Could you check a few things on this drawing? It's one solid part, dimensions in mm from its lowest x, y, z. Round coordinates to 2 decimals unless told otherwise and drop trailing zeros. Loops run counter-clockwise (first coordinate to the right, second up) from the corner with the lowest first, then second, coordinate; pieces in that order, holes last. Notation, with made-up numbers: M 56.25,-17 L 110.25,-17 A31 cw 110.25,21 Z; hole C 17.5,-14 d6. An arc over 180 degrees is marked long. Answer as a JSON object with one key per item and string values.
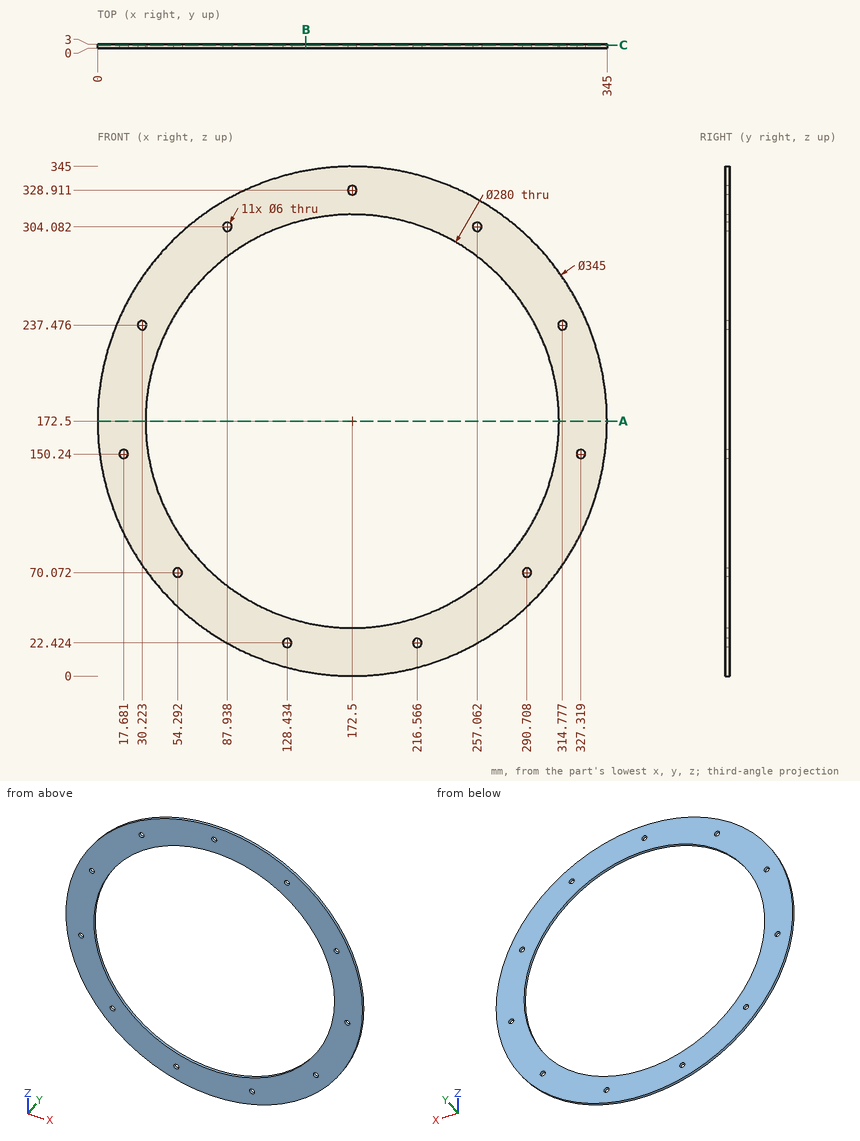
Item 1: I want a section at C-C, the plane y = 2.3. State how many separate pieces and enclosed holes the cut face has, then the cut area to 3 significant figures.
Resolved:
{"separate pieces": "1", "enclosed holes": "12", "area": "31,600 mm²"}
Item 2: I want a section at A-A, the plane z = 172.5. Please give me the cut outline in (x, y).
Resolved:
{"outline": "M 0,0 L 32.5,0 L 32.5,3 L 0,3 Z; M 312.5,0 L 345,0 L 345,3 L 312.5,3 Z"}
Item 3: I'm going to push a flat-ended pin straight in: pin 1 Ø1 at (y, z) = (2.5, 162) entering from +X. Where does the tip first touch, or does it pass through?
Resolved:
{"pin 1": "x = 344.71"}
Item 4: I want a section at B-B, the plane x = 141. Please give me the cut outline in (y, z), then the cut area to 3 significant figures.
Resolved:
{"outline": "M 0,2.9 L 3,2.9 L 3,36.09 L 0,36.09 Z; M 0,308.91 L 3,308.91 L 3,342.1 L 0,342.1 Z", "area": "199 mm²"}
Item 5: Please list where these lines run through material, in increasing order: probe 1 along Z at (x, y) = (129, 1.05) (1 decimal); probe 2 along Z at (x, y) = (172.5, 2.35); probe 3 along X at (y, z) = (0.2, 188). Write a range as from..to.
Resolved:
{"probe 1": "5.6..19.5, 25.4..39.4, 305.6..339.4", "probe 2": "0..32.5, 312.5..325.91, 331.91..345", "probe 3": "0.7..33.36, 311.64..344.3"}
